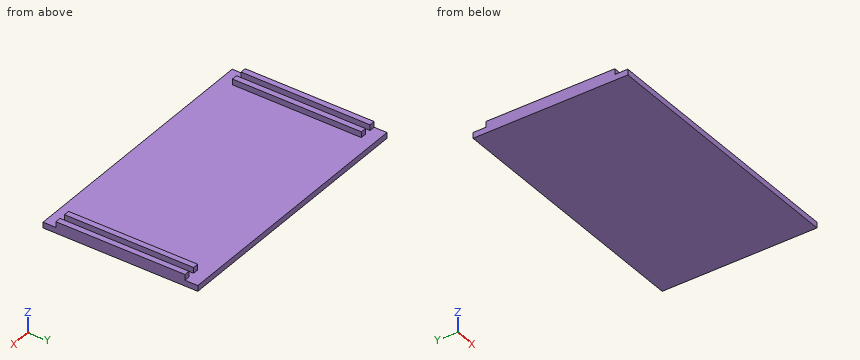
from build123d import *

# Parameters (mm, degrees)
BOSS_EXTRUDE1_DEPTH = 54
SKETCH7_W           = 185.5
SKETCH7_H           = 9
CUT_EXTRUDE4_DEPTH  = 4
SKETCH8_W           = 185.5
SKETCH8_H           = 9
CUT_EXTRUDE5_DEPTH  = 4


with BuildPart() as part:
    # Sketch1 → Boss-Extrude1 (new, symmetric)
    with BuildSketch(Plane(origin=(0, 0, 0), x_dir=(1, 0, 0), z_dir=(0, 1, 0))):
        Polygon((-63.408892702, 20.487993735), (122.091107298, 20.487993735), (122.091107298, 12.487993735), (118.091107298, 12.487993735), (118.091107298, 16.487993735), (113.591107298, 16.487993735), (113.591107298, 12.487993735), (109.591107298, 12.487993735), (109.591107298, 16.487993735), (-50.908892702, 16.487993735), (-50.908892702, 12.487993735), (-54.908892702, 12.487993735), (-54.908892702, 16.487993735), (-59.408892702, 16.487993735), (-59.408892702, 12.487993735), (-63.408892702, 12.487993735), align=None)
    extrude(amount=BOSS_EXTRUDE1_DEPTH, both=True)

    # Sketch7 → Cut-Extrude4 (cut)
    with BuildSketch(Plane.XY.offset(-12.487993735)):
        with Locations((29.341107298, 49.5)):
            Rectangle(SKETCH7_W, SKETCH7_H)
    extrude(amount=-CUT_EXTRUDE4_DEPTH, mode=Mode.SUBTRACT)

    # Sketch8 → Cut-Extrude5 (cut)
    with BuildSketch(Plane.XY.offset(-12.487993735)):
        with Locations((29.341107298, -49.5)):
            Rectangle(SKETCH8_W, SKETCH8_H)
    extrude(amount=-CUT_EXTRUDE5_DEPTH, mode=Mode.SUBTRACT)


solid = part.part
Check sheet for the modelled part. Datum: model origin and axes. Units: mm. Give positions to 0.01 mm unless a question says otherwise; leave off trailing zeros. Loops run counter-clockwise (first coordinate to the right, second up) from the corner with the lowest first, then second, coordinate; pieces in that order, holes last. Notation, with made-up numbers: M -17.75,-20 L 9.25,-20 A28 ccw 9.25,15 Z; hole C 44,4 d11. An arc over 180 degrees is marked long. Return JSON: item names as keys, results as strings. Group by question number.
1. Thickness scan on L1, parallel to X at y = -14.5, z = -14; L2, parallel to Z at x = 35, y = 13. Record the ranges inside material, lowest first.
2. Go/stop test with flat-tipped pins: pin 1 (2 mm diameter, centred on x = -53, z = -13.5, fed in from +Y); pin 2 (1.2 mm diameter, centred on x = 119.5, z = -15, fed in from -Y); pin 3 (8 mm diameter, centred on x = 78, y = 40, fed in from +Z). Record where each tip stops, or that it passes through.
3. Cross-section at B-B on y = 24. Record the boundary of the cut face in (x, z), plus the area to 3 significant figures.
4. Cross-section at C-C on x = -22. Record the boundary of the cut face in (y, z), plus the area to 3 significant figures.
5. Cross-section at A-A on z = -13.75. Record the boundary of the cut face in (x, y), plus the area to 3 significant figures.
Return value:
{
 "1": {"L1": "-63.41 to -59.41, -54.91 to -50.91, 109.59 to 113.59, 118.09 to 122.09", "L2": "-20.49 to -16.49"},
 "2": {"pin 1": "y = 45", "pin 2": "y = -45", "pin 3": "z = -16.49"},
 "3": {"outline": "M -63.41,-20.49 L 122.09,-20.49 L 122.09,-12.49 L 118.09,-12.49 L 118.09,-16.49 L 113.59,-16.49 L 113.59,-12.49 L 109.59,-12.49 L 109.59,-16.49 L -50.91,-16.49 L -50.91,-12.49 L -54.91,-12.49 L -54.91,-16.49 L -59.41,-16.49 L -59.41,-12.49 L -63.41,-12.49 Z", "area": "806 mm^2"},
 "4": {"outline": "M -54,-20.49 L 54,-20.49 L 54,-16.49 L -54,-16.49 Z", "area": "432 mm^2"},
 "5": {"outline": "M -63.41,-45 L -59.41,-45 L -59.41,45 L -63.41,45 Z; M -54.91,-45 L -50.91,-45 L -50.91,45 L -54.91,45 Z; M 109.59,-45 L 113.59,-45 L 113.59,45 L 109.59,45 Z; M 118.09,-45 L 122.09,-45 L 122.09,45 L 118.09,45 Z", "area": "1,440 mm^2"}
}
